```python
from build123d import *

# Parameters (mm, degrees)
ESBO_O1_W                  = 74
ESBO_O1_H                  = 77
RESSALTO_EXTRUS_O1_DEPTH   = 4
ESBO_O2_R                  = 13.5
CORTE_EXTRUS_O1_DEPTH      = 4
CORTE_EXTRUS_O1_DEPTH_BACK = 4
CORTE_EXTRUS_O2_DEPTH      = 1
CORTE_EXTRUS_O2_DEPTH_BACK = 5
FILETE2_R                  = 10
FILETE3_R                  = 10
FILETE4_R                  = 10


with BuildPart() as part:
    # Esboço1 → Ressalto-extrusão1 (new body)
    with BuildSketch(Plane.XY):
        with Locations((-49.165685596, 5.526315789)):
            Rectangle(ESBO_O1_W, ESBO_O1_H)
    extrude(amount=RESSALTO_EXTRUS_O1_DEPTH)

    # Esboço2 → Corte-extrusão1 (cut, two sides)
    with BuildSketch(Plane.XY.offset(4)) as corte_extrus_o1_sk:
        with Locations((-52.165685596, -2.973684211)):
            Circle(ESBO_O2_R)
    extrude(amount=CORTE_EXTRUS_O1_DEPTH, mode=Mode.SUBTRACT)
    extrude(corte_extrus_o1_sk.sketch, amount=-CORTE_EXTRUS_O1_DEPTH_BACK, mode=Mode.SUBTRACT)

    # Esboço4 → Corte-extrusão2 (cut, two sides)
    with BuildSketch(Plane.XY.offset(4)) as corte_extrus_o2_sk:
        Polygon((62.093925387, -180.88521739), (-61.165685596, -32.973684211), (-86.165685596, -2.973684211), (-209.425296578, 144.937848968), (-505.248362936, -101.581372997), (-233.729140971, -427.404439354), align=None)
    extrude(amount=CORTE_EXTRUS_O2_DEPTH, mode=Mode.SUBTRACT)
    extrude(corte_extrus_o2_sk.sketch, amount=-CORTE_EXTRUS_O2_DEPTH_BACK, mode=Mode.SUBTRACT)

    # Filete2
    filete2_edges = [part.edges().sort_by_distance(p)[0] for p in [
        (-86.165685596, -2.973684211, 2),
    ]]
    fillet(filete2_edges, radius=FILETE2_R)

    # Filete3
    filete3_edges = [part.edges().sort_by_distance(p)[0] for p in [
        (-61.165685596, -32.973684211, 2),
    ]]
    fillet(filete3_edges, radius=FILETE3_R)

    # Filete4
    filete4_edges = [part.edges().sort_by_distance(p)[0] for p in [
        (-12.165685596, 44.026315789, 2),
    ]]
    fillet(filete4_edges, radius=FILETE4_R)


solid = part.part
```
Input: part model. Units: mm. Frame: model coordinates. Give positions to 0.01 mm unless a question says otherwise; leave off trailing zeros. Loops run counter-clockwise (first coordinate to the right, second up) from the corner with the lowest first, then second, coordinate; pieces in that order, holes last.
1) Contact query for a flat-ended pin moving along its axis: pin 1 (21.5 mm diameter, centred on x = -52.17, y = -2.97, fed in from +Z). Output: stop coordinate, or through.
A:
pin 1: passes through
2) Mould query, pull axis Y, two halves, no side actions, for faces 1 (the flat face through (-55, 44.026, 2)), 2 (the cylindrical face through (-65.653, -2.38, 2.028)), 3 (the cylindrical face through (-85.585, -2.712, 1.972)). Classes: released by +Y, released by -Y, zero draft, split by the parting line, or undercut.
A:
face 1: released by +Y
face 2: undercut
face 3: released by -Y
3) Section query D-D on x = -80. Return the cut outline in (y, z), and give its area (3 significant figures).
A:
outline: (-10.37, 0) - (44.03, 0) - (44.03, 4) - (-10.37, 4) - close
area: 218 mm2
4) Section query A-A on y = 4. Return the cut outline in (x, z) (3 decimals), and give its area (3 significant figures).
A:
outline: (-86.166, 0) - (-63.725, 0) - (-63.725, 4) - (-86.166, 4) - close; (-40.606, 0) - (-12.166, 0) - (-12.166, 4) - (-40.606, 4) - close
area: 204 mm2
5) Section query B-B on x = -47. Return the cut outline in (y, z).
A:
outline: (-32.97, 0) - (-15.45, 0) - (-15.45, 4) - (-32.97, 4) - close; (9.5, 0) - (44.03, 0) - (44.03, 4) - (9.5, 4) - close
6) Section query C-C on z = 2.55. Return the cut outline in (x, y), and give its area (3 significant figures).
A:
outline: (-86.17, 0.65) arc R10 ccw to (-83.85, -5.76) - (-64.16, -29.38) arc R10 ccw to (-56.48, -32.97) - (-12.17, -32.97) - (-12.17, 34.03) arc R10 ccw to (-22.17, 44.03) - (-86.17, 44.03) - close; hole circle Ø27 at (-52.17, -2.97)
area: 4,720 mm2
7) Line query: L1, parallel to X at y = -11, z = 0.6; L2, parallel to X at y = -8.5, z = 2.4; L3, parallel to Y at x = -64, z = 1.85. Output: solid intervals per line, ascending.
A:
L1: x = -79.48 to -63.02, -41.31 to -12.17
L2: x = -81.56 to -64.48, -39.85 to -12.17
L3: y = -29.57 to -9.47, 3.52 to 44.03
